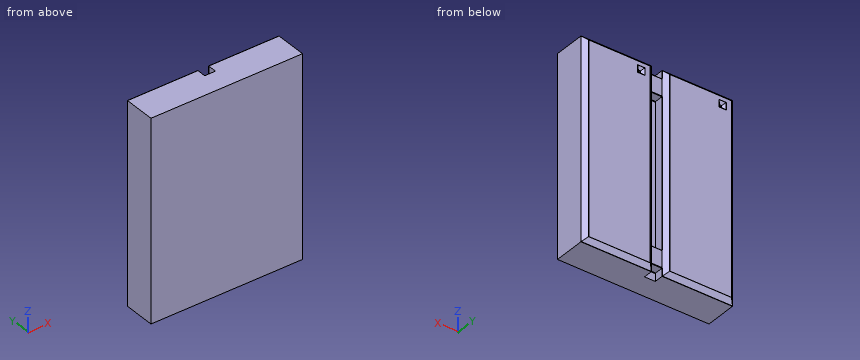
from build123d import *

# Parameters (mm, degrees)
SKETCH1_W           = 34.6
SKETCH1_H           = 45.6
BOSS_EXTRUDE1_DEPTH = 8.15
SKETCH2_W           = 2.47
SKETCH2_H           = 45.6
CUT_EXTRUDE1_DEPTH  = 3.09
CHAMFER1_SIZE       = 1
SKETCH3_W           = 2.47
SKETCH3_H           = 3.95
BOSS_EXTRUDE2_DEPTH = 2.09
SKETCH4_W           = 0.45
SKETCH4_H           = 0.45
CUT_EXTRUDE2_DEPTH  = 7.09
CHAMFER2_SIZE       = 0.6
FILLET2_R           = 0.05
FILLET3_R           = 0.1
FILLET4_R           = 0.1


with BuildPart() as part:
    # Sketch1 → Boss-Extrude1 (new body)
    with BuildSketch(Plane(origin=(0, 0, 0), x_dir=(1, 0, 0), z_dir=(0, 1, 0))):
        Rectangle(SKETCH1_W, SKETCH1_H)
    extrude(amount=BOSS_EXTRUDE1_DEPTH)

    # Sketch2 → Cut-Extrude1 (cut)
    with BuildSketch(Plane(origin=(0, 8.15, 0), x_dir=(1, 0, 0), z_dir=(0, 1, 0))):
        Rectangle(SKETCH2_W, SKETCH2_H)
    extrude(amount=-CUT_EXTRUDE1_DEPTH, mode=Mode.SUBTRACT)

    # Chamfer1
    chamfer1_edges = [part.edges().sort_by_distance(p)[0] for p in [
        (-17.3, 8.15, 0),
        (-9.2675, 8.15, 22.8),
        (-9.2675, 8.15, -22.8),
        (9.2675, 8.15, 22.8),
        (1.235, 8.15, 0),
        (-1.235, 8.15, 0),
        (17.3, 8.15, 0),
        (9.2675, 8.15, -22.8),
    ]]
    chamfer(chamfer1_edges, length=CHAMFER1_SIZE)

    # Sketch3 → Boss-Extrude2 (add)
    with BuildSketch(Plane(origin=(0, 5.06, 0), x_dir=(1, 0, 0), z_dir=(0, 1, 0))):
        with Locations((0, 19.005)):
            Rectangle(SKETCH3_W, SKETCH3_H)
        with Locations((0, -19.005)):
            Rectangle(SKETCH3_W, SKETCH3_H)
    extrude(amount=BOSS_EXTRUDE2_DEPTH)

    # Sketch4 → Cut-Extrude2 (cut)
    with BuildSketch(Plane(origin=(0, 8.15, 0), x_dir=(1, 0, 0), z_dir=(0, 1, 0))):
        with Locations((-14.275, -20.075)):
            Rectangle(SKETCH4_W, SKETCH4_H)
        with Locations((4.275, -20.075)):
            Rectangle(SKETCH4_W, SKETCH4_H)
    extrude(amount=-CUT_EXTRUDE2_DEPTH, mode=Mode.SUBTRACT)

    # Chamfer2
    chamfer2_edges = [part.edges().sort_by_distance(p)[0] for p in [
        (-14.05, 8.15, 20.075),
        (-14.275, 8.15, 19.85),
        (-14.5, 8.15, 20.075),
        (-14.275, 8.15, 20.3),
        (4.275, 8.15, 19.85),
        (4.05, 8.15, 20.075),
        (4.275, 8.15, 20.3),
        (4.5, 8.15, 20.075),
    ]]
    chamfer(chamfer2_edges, length=CHAMFER2_SIZE)

    # Fillet2
    fillet2_edges = [part.edges().sort_by_distance(p)[0] for p in [
        (2.235, 8.15, 0),
        (9.2675, 8.15, 21.8),
        (16.3, 8.15, 0),
        (9.2675, 8.15, -21.8),
        (-2.235, 8.15, 0),
        (-9.2675, 8.15, -21.8),
        (-16.3, 8.15, 0),
        (-9.2675, 8.15, 21.8),
        (3.45, 8.15, 20.075),
        (4.275, 8.15, 19.25),
        (5.1, 8.15, 20.075),
        (4.275, 8.15, 20.9),
        (-14.275, 8.15, 19.25),
        (-15.1, 8.15, 20.075),
        (-13.45, 8.15, 20.075),
        (-14.275, 8.15, 20.9),
    ]]
    fillet(fillet2_edges, radius=FILLET2_R)

    # Fillet3
    fillet3_edges = [part.edges().sort_by_distance(p)[0] for p in [
        (-9.2675, 7.15, -22.8),
        (9.2675, 7.15, -22.8),
        (17.3, 7.15, 0),
        (-9.2675, 7.15, 22.8),
        (9.2675, 7.15, 22.8),
        (1.235, 7.15, 21.89),
        (-17.3, 7.15, 0),
        (-1.235, 7.15, -21.89),
        (-1.235, 7.15, 0),
        (1.235, 7.15, -21.89),
        (-1.235, 7.15, 21.89),
        (1.235, 7.15, 0),
    ]]
    fillet(fillet3_edges, radius=FILLET3_R)

    # Fillet4
    fillet4_edges = [part.edges().sort_by_distance(p)[0] for p in [
        (0, 5.06, -20.98),
        (0, 5.06, -17.03),
        (0, 7.15, -20.98),
        (0, 7.15, -17.03),
        (0, 5.06, 17.03),
        (0, 5.06, 20.98),
        (0, 7.15, 17.03),
        (0, 7.15, 20.98),
    ]]
    fillet(fillet4_edges, radius=FILLET4_R)


solid = part.part
Could you check a few things on this model? Use its own coordinates, in mm. Coordinates: 2 decimals unless noted, no trailing zeros. Write each loop counter-clockwise with the first axis right and the second up, starting at its lowest first coordinate (ties: lowest second). Pieces come first, ordered by that corner, then holes. Notation, with made-up numbers: (3, 77) - (23, 77) arc R21 cw to (23, 88) - close; hole circle Ø11 at (33, -1.75). An arc over 180 degrees is marked (long way). Write item = value, one per line.
1) Please list where these lines run through material, in increasing order: line 1 (X direction, y = 7, z = 15) (3 decimals); line 2 (Y direction, x = -1, z = -5); line 3 (X direction, y = 7.5, z = -10) (3 decimals). Write a range as [from, to].
Result set:
line_1 = [-17.3, -1.235], [1.235, 17.3]
line_2 = [0, 5.06]
line_3 = [-16.95, -1.585], [1.585, 16.95]
2) Suppose I cut it at C-C on z = 18. Please give me the cut outline in (x, y) (3 decimals).
Result set:
outline = (-17.3, 0) - (17.3, 0) - (17.3, 7.109) arc R0.1 ccw to (17.271, 7.179) - (16.315, 8.135) arc R0.05 ccw to (16.279, 8.15) - (2.256, 8.15) arc R0.05 ccw to (2.22, 8.135) - (1.235, 7.15) - (-1.235, 7.15) - (-2.22, 8.135) arc R0.05 ccw to (-2.256, 8.15) - (-16.279, 8.15) arc R0.05 ccw to (-16.315, 8.135) - (-17.271, 7.179) arc R0.1 ccw to (-17.3, 7.109) - close
3) Will these pins go through, and if not, where does the flat tip stop? pin 1 Ø1 at (x, y) = (0.5, 6) entering from -Z; pin 2 Ø0.7 at (x, z) = (0.5, 20) entering from +Y; pin 3 Ø0.5 at (x, z) = (-14, 20) entering from +Y.
Result set:
pin_1 = -20.98
pin_2 = 7.15
pin_3 = 7.85
4) Suppose I cut it at B-B on y = 6.5. Please give me the cut outline in (x, z) (3 decimals), plus the area to 3 significant figures.
Result set:
outline = (-17.3, -22.8) - (-1.235, -22.8) - (-1.235, -20.98) - (1.235, -20.98) - (1.235, -22.8) - (17.3, -22.8) - (17.3, 22.8) - (1.235, 22.8) - (1.235, 20.98) - (-1.235, 20.98) - (-1.235, 22.8) - (-17.3, 22.8) - close; hole (-14.5, 19.85) - (-14.05, 19.85) - (-14.05, 20.3) - (-14.5, 20.3) - close; hole (-1.235, -17.03) - (1.235, -17.03) - (1.235, 17.03) - (-1.235, 17.03) - close; hole (4.05, 19.85) - (4.5, 19.85) - (4.5, 20.3) - (4.05, 20.3) - close
area = 1,480 mm2
5) Suppose I cut it at A-A on z = -4. Please give me the cut outline in (x, y) (3 decimals), plus the area to 3 significant figures.
Result set:
outline = (-17.3, 0) - (17.3, 0) - (17.3, 7.109) arc R0.1 ccw to (17.271, 7.179) - (16.315, 8.135) arc R0.05 ccw to (16.279, 8.15) - (2.256, 8.15) arc R0.05 ccw to (2.22, 8.135) - (1.264, 7.179) arc R0.1 ccw to (1.235, 7.109) - (1.235, 5.06) - (-1.235, 5.06) - (-1.235, 7.109) arc R0.1 ccw to (-1.264, 7.179) - (-2.22, 8.135) arc R0.05 ccw to (-2.256, 8.15) - (-16.279, 8.15) arc R0.05 ccw to (-16.315, 8.135) - (-17.271, 7.179) arc R0.1 ccw to (-17.3, 7.109) - close
area = 272 mm2
